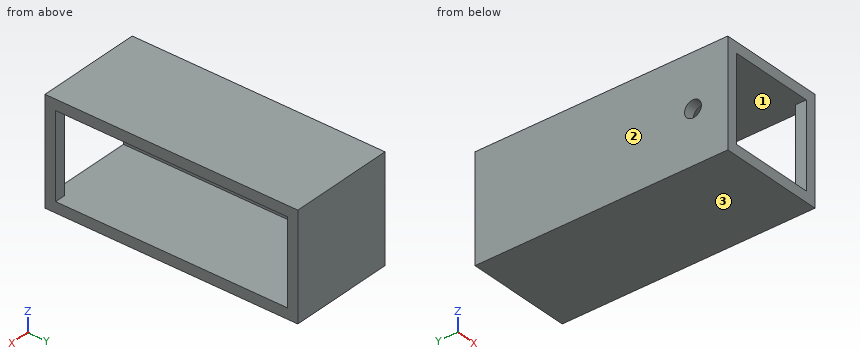
```python
from build123d import *

# Parameters (mm, degrees)
F0_W     = 250
F0_H     = 250
F1_DEPTH = 600
F2_W     = 200
F2_H     = 200
F3_DEPTH = 575
F4_W     = 550
F4_H     = 200
F5_DEPTH = 48
F7_D     = 40
F7_DEPTH = 25


with BuildPart() as f1:
    # F0 (on Front) → F1 (new body)
    with BuildSketch(Plane.XZ):
        Rectangle(F0_W, F0_H)
    extrude(amount=-F1_DEPTH)

    # F2 (on face) → F3 (cut)
    with BuildSketch(Plane.XZ):
        Rectangle(F2_W, F2_H)
    extrude(amount=-F3_DEPTH, mode=Mode.SUBTRACT)

    # F4 (on face) → F5 (cut)
    with BuildSketch(Plane.YZ.offset(125)):
        with Locations((300, 0)):
            Rectangle(F4_W, F4_H)
    extrude(amount=-F5_DEPTH, mode=Mode.SUBTRACT)

    # F7
    with Locations(Plane(origin=(-125, 0, 0), x_dir=(0, -1, 0), z_dir=(-1, 0, 0))):
        with Locations((-82.651734, 0)):
            Hole(F7_D / 2, depth=F7_DEPTH)


solid = f1.part
```
For this review, take the finished solid that the model builds, in its own axes (mm). Face numbers are marked on the shaded views. Round coordinates to 2 decimals unless told otherwise and drop trailing zeros. Write each loop counter-clockwise with the first axis right and the second up, starting at its lowest first coordinate (ties: lowest second). Pieces come first, ordered by that corner, then holes. Notation, with made-up numbers: (31.25, -17) -> (58.25, -17) arc R21 ccw to (58.25, 0) -> close; hole circle Ø6 at (2, 42). An arc over 180 degrees is marked (long way). Use one line per item in the form item = value.
1) Take a section at A-A, the plane z = -32. Write out the cut boundary in (x, y), and give its area (4 significant figures).
Found:
outline = (-125, 0) -> (-100, 0) -> (-100, 575) -> (125, 575) -> (125, 600) -> (-125, 600) -> close; (100, 0) -> (125, 0) -> (125, 25) -> (100, 25) -> close
area = 21,250 mm2
2) Take a section at D-D, the plane y = 296.5. Write out the cut boundary in (x, z), and give its area (3 significant figures).
Found:
outline = (-125, -125) -> (125, -125) -> (125, -100) -> (-100, -100) -> (-100, 100) -> (125, 100) -> (125, 125) -> (-125, 125) -> close
area = 17,500 mm2
3) Take a section at B-B, the plane z = 0. Write out the cut boundary in (x, y).
Found:
outline = (-125, 0) -> (-100, 0) -> (-100, 62.65) -> (-125, 62.65) -> close; (-125, 102.65) -> (-100, 102.65) -> (-100, 575) -> (125, 575) -> (125, 600) -> (-125, 600) -> close; (100, 0) -> (125, 0) -> (125, 25) -> (100, 25) -> close
4) To check wall thickness, follow L1, parallel to Z at x = 99, y = 449.5; L2, parallel to Y at x = 104.5, z = 66; L3, parallel to X at y = 268, z = -63.5. State the ranges of each line that lie inside material, in increasing order. Write a range as from..to.
Found:
L1 = -125..-100, 100..125
L2 = 0..25, 575..600
L3 = -125..-100
5) Take a section at C-C, the plane x = -91. Write out the cut boundary in (y, z), and give its area (3 significant figures).
Found:
outline = (0, -125) -> (600, -125) -> (600, 125) -> (0, 125) -> (0, 100) -> (575, 100) -> (575, -100) -> (0, -100) -> close
area = 35,000 mm2
6) Mouldability with a two-part tool opening along Z and no side actions: class the marked faces 1, 2 and 3 as +Z half, -Z half, draft (parallel to the pull), parting line (faces both ways), or undercut.
Found:
face_1 = undercut
face_2 = draft
face_3 = -Z half
7) Clearance check with flat-ended pins moving along their axes: pin 1 (6 mm diameter, centred on x = -2, z = 24.5, fed in from -Y); pin 2 (12 mm diameter, centred on y = 532.5, z = 67, fed in from +X). State where each tip first meets the part, or that it passes through.
Found:
pin_1 = 575
pin_2 = -100
